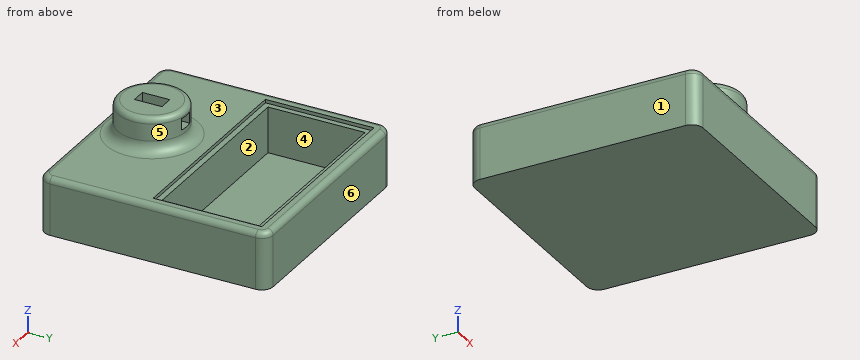
```python
from build123d import *

# Parameters (mm, degrees)
SKICA1_W                 = 200.00000000000003
SKICA1_H                 = 200.00000000000003
P_IDAT_VYSUNUT_M3_DEPTH  = 50
ZAOBLIT1_R               = 10
SKICA2_R                 = 29.999999999999996
P_IDAT_VYSUNUT_M4_DEPTH  = 30
ZAOBLIT2_R               = 10
ZAOBLIT3_R               = 5
ODEBRAT_VYSUNUT_M1_DEPTH = 3
ODEBRAT_VYSUNUT_M2_DEPTH = 40
ZAOBLIT5_R               = 5
ODEBRAT_VYSUNUT_M3_DEPTH = 16
SKICA10_W                = 12.699999999999989
SKICA10_H                = 10
ODEBRAT_VYSUNUT_M4_DEPTH = 259.5517356352496


with BuildPart() as part:
    # Skica1 → Přidat vysunutím3 (new body)
    with BuildSketch(Plane.XY):
        with Locations((100.00000000000001, 100.00000000000001)):
            Rectangle(SKICA1_W, SKICA1_H)
    extrude(amount=P_IDAT_VYSUNUT_M3_DEPTH)

    # Zaoblit1
    zaoblit1_edges = [part.edges().sort_by_distance(p)[0] for p in [
        (0, 200, 25),
        (200, 200, 25),
        (200, 0, 25),
        (0, 0, 25),
    ]]
    fillet(zaoblit1_edges, radius=ZAOBLIT1_R)

    # Skica2 → Přidat vysunutím4 (add)
    with BuildSketch(Plane.XY.offset(50)):
        with Locations(Location((100, 45.000000000000014, 0), (0, 0, 180))):
            Circle(SKICA2_R)
    extrude(amount=P_IDAT_VYSUNUT_M4_DEPTH)

    # Zaoblit2
    zaoblit2_edges = [part.edges().sort_by_distance(p)[0] for p in [
        (130, 45.00000000000001, 50),
    ]]
    fillet(zaoblit2_edges, radius=ZAOBLIT2_R)

    # Zaoblit3
    zaoblit3_edges = [part.edges().sort_by_distance(p)[0] for p in [
        (130, 45.00000000000001, 80),
    ]]
    fillet(zaoblit3_edges, radius=ZAOBLIT3_R)

    # Skica4 → Odebrat vysunutím1 (cut)
    with BuildSketch(Plane.XY.offset(50)):
        Polygon((10, 190), (190, 190), (190, 95.00000000000001), (10.000000000000012, 95.00000000000001), align=None)
    extrude(amount=-ODEBRAT_VYSUNUT_M1_DEPTH, mode=Mode.SUBTRACT)

    # Skica7 → Odebrat vysunutím2 (cut)
    with BuildSketch(Plane.XY.offset(47)):
        Polygon((14.999999999999998, 185), (185, 185), (185, 100.00000000000001), (15.00000000000001, 100.00000000000001), align=None)
    extrude(amount=-ODEBRAT_VYSUNUT_M2_DEPTH, mode=Mode.SUBTRACT)

    # Zaoblit5
    zaoblit5_edges = [part.edges().sort_by_distance(p)[0] for p in [
        (200, 100, 50),
        (100, 0, 50),
        (0, 100, 50),
        (100, 200, 50),
        (2.9289321881345236, 2.9289321881345227, 50),
        (2.9289321881345236, 197.07106781186548, 50),
        (197.07106781186548, 197.07106781186548, 50),
        (197.07106781186548, 2.9289321881345236, 50),
    ]]
    fillet(zaoblit5_edges, radius=ZAOBLIT5_R)

    # Skica9 → Odebrat vysunutím3 (cut)
    with BuildSketch(Plane.XY.offset(80)):
        Polygon((99.99999999999999, 45.000000000000014), (93.64999999999999, 57.000000000000014), (93.64999999999999, 45.000000000000014), align=None)
        Polygon((100, 57.000000000000014), (93.64999999999999, 57.000000000000014), (99.99999999999999, 45.000000000000014), align=None)
        Polygon((100, 57.000000000000014), (100, 45.00000000000002), (106.35, 57.000000000000014), align=None)
        Polygon((106.35, 57.000000000000014), (100, 45.00000000000003), (106.35, 45.000000000000014), align=None)
        Polygon((106.35, 45.000000000000014), (100, 45.000000000000014), (106.35, 33.000000000000014), align=None)
        Polygon((106.35, 33.000000000000014), (99.99999999999999, 45.000000000000014), (100, 33.000000000000014), align=None)
        Polygon((100, 33.000000000000014), (100, 45.00000000000002), (93.64999999999999, 33.000000000000014), align=None)
        Polygon((93.64999999999999, 33.000000000000014), (100, 45.00000000000003), (93.64999999999999, 45.000000000000014), align=None)
    extrude(amount=-ODEBRAT_VYSUNUT_M3_DEPTH, mode=Mode.SUBTRACT)

    # Skica10 → Odebrat vysunutím4 (cut, through all)
    with BuildSketch(Plane(origin=(0, 57.000000000000014, 0), x_dir=(-1, 0, 0), z_dir=(0, -1, 0))):
        with Locations((-99.99999999999999, -69)):
            Rectangle(SKICA10_W, SKICA10_H)
    extrude(amount=-ODEBRAT_VYSUNUT_M4_DEPTH, mode=Mode.SUBTRACT)


solid = part.part
```
For this review, take the finished solid that the model builds, in its own axes (mm). Face numbers are marked on the shaded views. A direction names the side the tool comes from. Give positions to 0.01 mm unless a question says otherwise; leave off trailing zeros. Order: outer loops, then holes, each group sorted by start corner. A loop starts at its lowest first (then second) coordinate and runs counter-clockwise, first axis right, second up.
1) Wall thickness on line 1 (Y direction, x = 97.5, z = 33.5); line 2 (X direction, y = 141, z = 35); line 3 (Z direction, x = 60, y = 71): over which ranges is each line inside the solid? List them lowest first.
2) Take a section at C-C (z = 70). Give the boundary of the cut face in (x, y).
3) The part is to be moulded in two halves that separate along X. For the marked faces 1, 2, 3 and 4, say which applies: released by +X, released by -X, zero draft, split by the parting line, or undercut.
4) Take a section at B-B (y = 108.5). Give the boundary of the cut face in (x, z).
5) Insertion check: pin 1 (1.5 mm diameter, centred on x = 134, y = 44.5, fed in from -Z); pin 2 (13 mm diameter, centred on y = 55, z = 74, fed in from +X); pin 3 (3 mm diameter, centred on y = 104, z = 49.5, fed in from -X); pin 4 (1.5 mm diameter, centred on x = 106, z = 49, fed in from -Y). Each pin has a flat end and moves straight along its axis. Give the tip position at first contact, or say it passes through.
6) For the marked faces 5 and 6, list the 3-axis set-ups (+Z, -Z, +X, -X, +Y, -Y) from which the entire face can be reached by the end or side of a thin tool; tool diameter is ignored.
7) Take a section at A-A (x = 32). Give the boundary of the cut face in (y, z), then the cut area to 3 significant figures.
Derived:
1. line 1: y = 0 to 100, 185 to 200
1. line 2: x = 0 to 15, 185 to 200
1. line 3: z = 0 to 50
2. outline: (93.65, 33) - (93.65, 74.32) arc R30 ccw (long way) to (106.35, 74.32) - (106.35, 33) - close
3. face 1: released by -X
3. face 2: undercut
3. face 3: zero draft
3. face 4: undercut
4. outline: (0, 0) - (200, 0) - (200, 45) arc R5 ccw to (195, 50) - (190, 50) - (190, 47) - (185, 47) - (185, 7) - (15, 7) - (15, 47) - (10, 47) - (10, 50) - (5, 50) arc R5 ccw to (0, 45) - close
5. pin 1: stops at z = 0
5. pin 2: stops at x = 129.8
5. pin 3: stops at x = 1
5. pin 4: stops at y = 1.2
6. face 5: +Z
6. face 6: +Z, -Z, +X, -X, +Y
7. outline: (0, 0) - (200, 0) - (200, 45) arc R5 ccw to (195, 50) - (190, 50) - (190, 47) - (185, 47) - (185, 7) - (100, 7) - (100, 47) - (95, 47) - (95, 50) - (5, 50) arc R5 ccw to (0, 45) - close
7. area: 6,300 mm2
